Part model, mm, in its own coordinate system. A direction names the side the tool comes from. Round coordinates to 2 decimals unless told otherwise and drop trailing zeros. Order: outer loops, then holes, each group sorted by start corner. A loop starts at its lowest first (then second) coordinate and runs counter-clockwise, first axis right, second up. Notation, with made-up numbers: (82.5, -25) - (93.5, -25) arc R19 cw to (93.5, -4) - close; hole circle Ø4 at (2, 84.5). An arc over 180 degrees is marked (long way). Answer as a JSON object with one key per item and string values.
```python
from build123d import *

# Parameters (mm, degrees)
SKETCH1_W           = 18
SKETCH1_H           = 18
SKETCH3_W           = 54
SKETCH3_H           = 18
BOSS_EXTRUDE1_DEPTH = 10.16
SKETCH4_W           = 8
SKETCH4_H           = 8
SKETCH6_R           = 2.125
CUT_EXTRUDE1_DEPTH  = 136.095622661
SKETCH7_R           = 3.3
CUT_EXTRUDE2_DEPTH  = 3
SKETCH8_W           = 4
SKETCH8_H           = 20
CUT_EXTRUDE3_DEPTH  = 2
SKETCH9_W           = 18
SKETCH9_H           = 18
BOSS_EXTRUDE2_DEPTH = 20.32
SKETCH10_R          = 1.6764
CUT_EXTRUDE4_DEPTH  = 15.24


with BuildPart() as part:
    # Sweep1: sweep along a path in Sketch2
    with BuildLine(Plane.XY) as sweep1_path:
        Line((-10.900401277, 0), (16.094282055, 127))
    # Sketch1 → Sweep1 (sweep)
    with BuildSketch(Plane(origin=(0, 0, 0), x_dir=(1, 0, 0), z_dir=(0, 1, 0))):
        with Locations((-1.900401277, 0.398563086)):
            Rectangle(SKETCH1_W, SKETCH1_H)
    sweep(path=sweep1_path.line)

    # Sketch3 → Boss-Extrude1 (add)
    with BuildSketch(Plane(origin=(0, 127, 0), x_dir=(1, 0, 0), z_dir=(0, 1, 0))):
        with Locations((18.094282055, 0.398563086)):
            Rectangle(SKETCH3_W, SKETCH3_H)
    extrude(amount=BOSS_EXTRUDE1_DEPTH)

    # Cut-Sweep1: sweep along a path in Sketch5
    with BuildLine(Plane.XY.offset(8.601436914)) as cut_sweep1_path:
        Line((-5.900401277, 0), (9.942469563, 74.534847176))
    # Sketch4 → Cut-Sweep1 (sweep, cut)
    with BuildSketch(Plane.XZ):
        with Locations((-1.900401277, -0.398563086)):
            Rectangle(SKETCH4_W, SKETCH4_H)
    sweep(path=cut_sweep1_path.line, mode=Mode.SUBTRACT)

    # Sketch6 → Cut-Extrude1 (cut, through all)
    with BuildSketch(Plane.XZ.offset(-127)):
        with Locations(Location((37.894282055, -0.398563086, 0), (0, 0, 270))):
            Circle(SKETCH6_R)
        with Locations(Location((11.794282055, -0.398563086, 0), (0, 0, 270))):
            Circle(SKETCH6_R)
    extrude(amount=-CUT_EXTRUDE1_DEPTH, mode=Mode.SUBTRACT)

    # Sketch7 → Cut-Extrude2 (cut)
    with BuildSketch(Plane.XZ.offset(-127)):
        with Locations(Location((11.794282055, -0.398563086, 0), (0, 0, 270))):
            Circle(SKETCH7_R)
        with Locations(Location((37.894282055, -0.398563086, 0), (0, 0, 270))):
            Circle(SKETCH7_R)
    extrude(amount=-CUT_EXTRUDE2_DEPTH, mode=Mode.SUBTRACT)

    # Sketch8 → Cut-Extrude3 (cut)
    with BuildSketch(Plane(origin=(-10.429206675, 2.216796312, 0), x_dir=(0, 0, 1), z_dir=(-0.9781476007338064, 0.20791169081775596, 0))):
        with Locations((-0.398563086, 117.570934688)):
            Rectangle(SKETCH8_W, SKETCH8_H)
    extrude(amount=-CUT_EXTRUDE3_DEPTH, mode=Mode.SUBTRACT)

    # Sketch9 → Boss-Extrude2 (add)
    with BuildSketch(Plane.XZ):
        with Locations((-1.900401277, -0.398563086)):
            Rectangle(SKETCH9_W, SKETCH9_H)
    extrude(amount=BOSS_EXTRUDE2_DEPTH)

    # Sketch10 → Cut-Extrude4 (cut)
    with BuildSketch(Plane.XZ.offset(20.32)):
        with Locations(Location((-1.900401277, -0.398563086, 0), (0, 0, 270))):
            Circle(SKETCH10_R)
    extrude(amount=-CUT_EXTRUDE4_DEPTH, mode=Mode.SUBTRACT)


solid = part.part
```
Item 1: Cut at A-A (z = 5.75). Write the cut outline in (x, y).
Taken from the geometry:
{"outline": "(-10.9, -20.32) - (7.1, -20.32) - (7.1, 0) - (34.09, 127) - (45.09, 127) - (45.09, 137.16) - (-8.91, 137.16) - (-8.91, 127) - (16.09, 127) - (-10.9, 0) - close"}
Item 2: Cut at B-B (y = 48). Write the cut outline in (x, z).
Taken from the geometry:
{"outline": "(-0.7, -9.4) - (17.3, -9.4) - (17.3, 8.6) - (-0.7, 8.6) - close; hole (4.3, -4.4) - (12.3, -4.4) - (12.3, 3.6) - (4.3, 3.6) - close"}
Item 3: Drop flat-ended pins along their axis: P1, Ø5.5, axis at y = -13.5, z = 3, coming from the +X side; P2, Ø10, axis at y = 97, z = 2, coming from the -X side; P3, Ø8, axis at y = 120.5, z = -4.5, coming from the -X side. Give the stop position or say it passes through.
Taken from the geometry:
{"P1": "x = 7.1", "P2": "x = 8.65", "P3": "x = 13.86"}
Item 4: Cut at D-D (x = 25). Write the cut outline in (y, z), plus the area to 3 significant figures.
Taken from the geometry:
{"outline": "(84.21, -9.4) - (137.16, -9.4) - (137.16, 8.6) - (84.21, 8.6) - close", "area": "953 mm2"}
Item 5: Tool access for faces 4 (the flat face through (38, 130, -3)), 5 (the flat face through (45.094, 132, 0)), 6 (the flat face through (7.1, -10, -1)), 7 (the flat face through (2.132, 37.789, -0.343)), 8 (the flat face through (-8.906, 132, 0)): list every direction of +Z, -Z, +X, -X, +Y, -Y with a clear straight run to the whole face (end or side of a thin tool).
Taken from the geometry:
{"face 4": "-Y", "face 5": "+Z, -Z, +X, +Y, -Y", "face 6": "+Z, -Z, +X, -Y", "face 7": "none", "face 8": "+Z, -Z, -X, +Y"}
Item 6: Probe L1, parallel to Z at x = 15, y = 121; L2, parallel to Z at x = -0.5, y = 17.5; L3, parallel to X at y = -1, z = -5. List the from-to ranges inside material, lowest first. Write a range as from..to.
Taken from the geometry:
{"L1": "-9.4..-2.4, 1.6..8.6", "L2": "-9.4..-4.4, 3.6..8.6", "L3": "-10.9..7.1"}
Item 7: Cut at C-C (z = -0.5). State how many separate pieces and enclosed holes the cut face has, plus the area to 3 significant figures.
Taken from the geometry:
{"separate pieces": "3", "enclosed holes": "1", "area": "2,410 mm2"}
Item 8: Two-plate mould, pull along Z, no slides. Class faces 1 (the flat face through (15, 117, -2.399)), 2 (the flat face through (0, -20.32, 0)), 3 (the flat face through (10, 77, 8.601)): pulls with the +Z half, pulls with the -Z half, needs draft (parallel to the pull), parting line crosses it, or undercut.
Taken from the geometry:
{"face 1": "undercut", "face 2": "needs draft", "face 3": "pulls with the +Z half"}
